from build123d import *

# Parameters (mm, degrees)
SKETCH1_W           = 20
SKETCH1_H           = 3
SKETCH1_W_2         = 50
SKETCH1_H_2         = 40
BOSS_EXTRUDE1_DEPTH = 3.9


with BuildPart() as part:
    # Sketch1 → Boss-Extrude1 (new body)
    with BuildSketch(Plane(origin=(0, 0, 0), x_dir=(1, 0, 0), z_dir=(0, 1, 0))):
        Polygon((-125, 75), (-100, 75), (-100, 71.1), (-80, 71.1), (-80, 75), (-10, 75), (-10, 71.1), (10, 71.1), (10, 75), (80, 75), (80, 71.1), (100, 71.1), (100, 75), (125, 75), (125, 50), (121.1, 50), (121.1, 30), (125, 30), (125, -30), (121.1, -30), (121.1, -50), (125, -50), (125, -75), (100, -75), (100, -71.1), (80, -71.1), (80, -75), (10, -75), (10, -71.1), (-10, -71.1), (-10, -75), (-80, -75), (-80, -71.1), (-100, -71.1), (-100, -75), (-125, -75), (-125, -50), (-121.1, -50), (-121.1, -30), (-125, -30), (-125, 30), (-121.1, 30), (-121.1, 50), (-125, 50), align=None)
        with Locations((-55, -50.5)):
            Rectangle(SKETCH1_W, SKETCH1_H, mode=Mode.SUBTRACT)
        with Locations((-55, -59.5)):
            Rectangle(SKETCH1_W, SKETCH1_H, mode=Mode.SUBTRACT)
        Rectangle(SKETCH1_W_2, SKETCH1_H_2, mode=Mode.SUBTRACT)
        with Locations((55, -59.5)):
            Rectangle(SKETCH1_W, SKETCH1_H, mode=Mode.SUBTRACT)
        with Locations((55, -50.5)):
            Rectangle(SKETCH1_W, SKETCH1_H, mode=Mode.SUBTRACT)
        with Locations((55, 50.5)):
            Rectangle(SKETCH1_W, SKETCH1_H, mode=Mode.SUBTRACT)
        with Locations((55, 59.5)):
            Rectangle(SKETCH1_W, SKETCH1_H, mode=Mode.SUBTRACT)
        with Locations((-55, 59.5)):
            Rectangle(SKETCH1_W, SKETCH1_H, mode=Mode.SUBTRACT)
        with Locations((-55, 50.5)):
            Rectangle(SKETCH1_W, SKETCH1_H, mode=Mode.SUBTRACT)
    extrude(amount=BOSS_EXTRUDE1_DEPTH)


solid = part.part
Build history of the part. All positions in model axes, mm. Round coordinates to 2 decimals unless told otherwise and drop trailing zeros. Write each loop counter-clockwise with the first axis right and the second up, starting at its lowest first coordinate (ties: lowest second). Pieces come first, ordered by that corner, then holes. Notation, with made-up numbers: M -0.5,20.25 L 52.5,20.25 A23 cw 52.5,49.25 Z; hole C 21.5,-21.5 d2. An arc over 180 degrees is marked long. Answer as a JSON object with one key per item and string values. Group by question number.
(1) Cut at B-B (z = -17.5). Give the cut face in (x, y).
(2) Cut at C-C (y = 1.65). Give the number of separate pieces and of enclosed holes in the cut face, and give its area (3 significant figures).
(3) Cut at A-A (x = -47.5). Give the cut face in (y, z).
(4) Cut at D-D (z = -35.5). Give the cut face in (x, y).
(5) Drill centre lines: L1, parallel to X at y = 1.4, z = -49.5; L2, parallel to Z at x = -50, y = 3.25; L3, parallel to Z at x = 3, y = 0.75. Where is each one in solid material? Low to high.
Responses:
{
 "1": {"outline": "M -125,0 L -25,0 L -25,3.9 L -125,3.9 Z; M 25,0 L 125,0 L 125,3.9 L 25,3.9 Z"},
 "2": {"separate pieces": "1", "enclosed holes": "9", "area": "34,200 mm2"},
 "3": {"outline": "M 0,-75 L 3.9,-75 L 3.9,-61 L 0,-61 Z; M 0,-58 L 3.9,-58 L 3.9,-52 L 0,-52 Z; M 0,-49 L 3.9,-49 L 3.9,49 L 0,49 Z; M 0,52 L 3.9,52 L 3.9,58 L 0,58 Z; M 0,61 L 3.9,61 L 3.9,75 L 0,75 Z"},
 "4": {"outline": "M -121.1,0 L 121.1,0 L 121.1,3.9 L -121.1,3.9 Z"},
 "5": {"L1": "x = -121.1 to -65, -45 to 45, 65 to 121.1", "L2": "z = -75 to -61, -58 to -52, -49 to 49, 52 to 58, 61 to 75", "L3": "z = -71.1 to -20, 20 to 71.1"}
}
